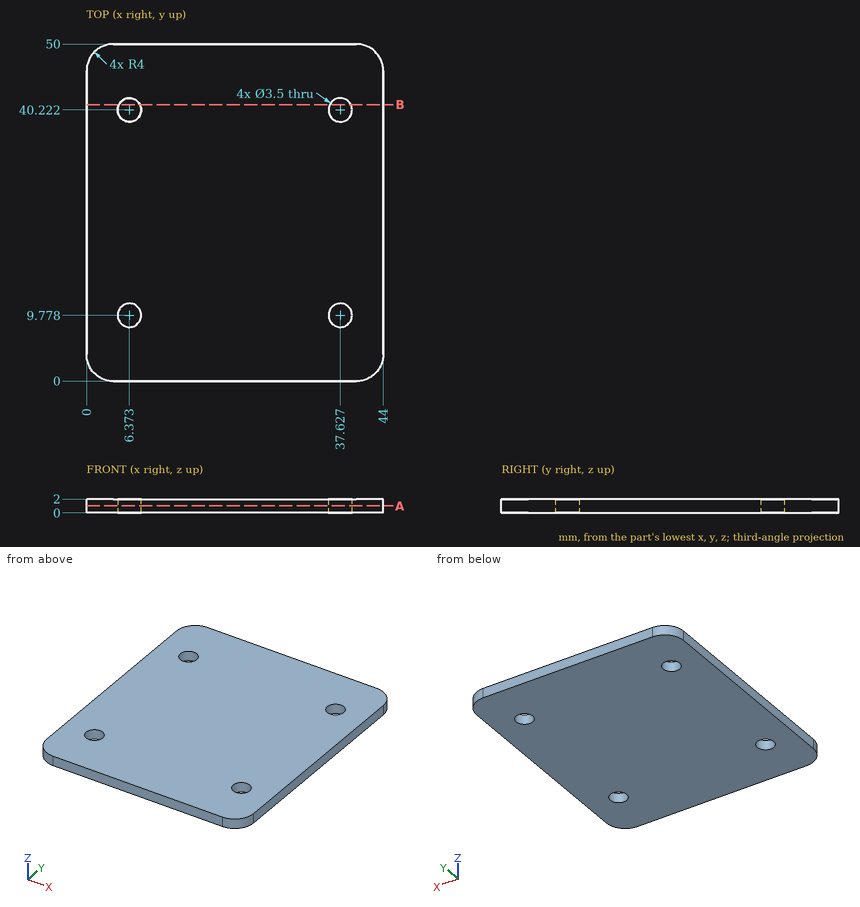
Geometry: see drawing. Coordinates: mm, zero at the bounding-box minimum. Round coordinates to 2 decimals unless told otherwise and drop trailing zeros. Write each loop counter-clockwise with the first axis right and the second up, starting at its lowest first coordinate (ties: lowest second). Pieces come first, ordered by that corner, then holes. Notation, with made-up numbers: (11.5, -18) - (57.5, -18) arc R11 cw to (57.5, -4) - close; hole circle Ø8 at (-8.75, 5.25). An arc over 180 degrees is marked (long way). Use CSV: the item, a comma, the result in double quotes. Start each with the question number.
(1) Cut plane B-B, the plane y = 41. Return loops of the section in (x, z) (1 decimal).
(2) Material intervals for probe 1 along Y at (x, z) = (5, 0.4); probe 2 along Y at (x, z) = (38.5, 0.55) (1 decimal); probe 3 along X at (y, z) = (9.5, 1.3) (1 decimal), sorted ascending. Write a range as [from, to].
(3) Cut plane A-A, the plane z = 1. Return loops of the section in (x, y), and give its area (3 significant figures).
Geometry says:
1,outline,"(0, 0) - (4.8, 0) - (4.8, 2) - (0, 2) - close; (7.9, 0) - (36.1, 0) - (36.1, 2) - (7.9, 2) - close; (39.2, 0) - (44, 0) - (44, 2) - (39.2, 2) - close"
2,probe 1,"[0, 8.69], [10.86, 39.14], [41.31, 50]"
2,probe 2,"[0, 8.3], [11.3, 38.7], [41.7, 50]"
2,probe 3,"[0, 4.6], [8.1, 35.9], [39.4, 44]"
3,outline,"(0, 4) arc R4 ccw to (4, 0) - (40, 0) arc R4 ccw to (44, 4) - (44, 46) arc R4 ccw to (40, 50) - (4, 50) arc R4 ccw to (0, 46) - close; hole circle Ø3.5 at (6.37, 9.78); hole circle Ø3.5 at (6.37, 40.22); hole circle Ø3.5 at (37.63, 9.78); hole circle Ø3.5 at (37.63, 40.22)"
3,area,"2,150 mm²"
